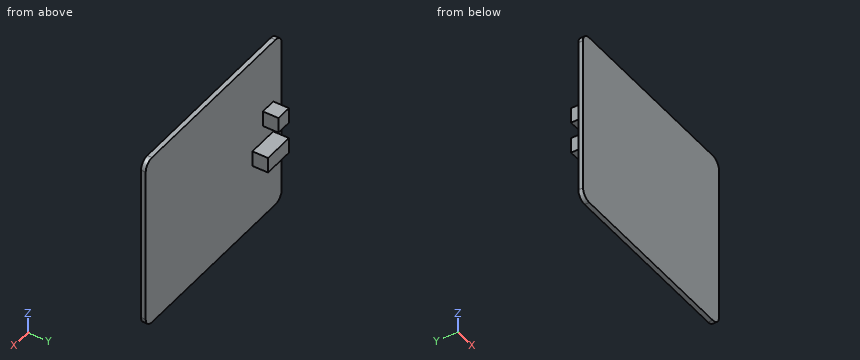
from build123d import *

# Parameters (mm, degrees)
SKETCH1_W           = 65
SKETCH1_H           = 56.6
BOSS_EXTRUDE1_DEPTH = 1.5
FILLET1_R           = 3
SKETCH2_W           = 5
SKETCH2_H           = 5
SKETCH2_W_2         = 10
BOSS_EXTRUDE2_DEPTH = 5


with BuildPart() as part:
    # Sketch1 → Boss-Extrude1 (new body)
    with BuildSketch(Plane(origin=(0, 0, 0), x_dir=(1, 0, 0), z_dir=(0, 1, 0))):
        with Locations((32.5, 28.3)):
            Rectangle(SKETCH1_W, SKETCH1_H)
    extrude(amount=BOSS_EXTRUDE1_DEPTH)

    # Fillet1
    fillet1_edges = [part.edges().sort_by_distance(p)[0] for p in [
        (0, 0.75, -56.6),
        (65, 0.75, -56.6),
        (65, 0.75, 0),
        (0, 0.75, 0),
    ]]
    fillet(fillet1_edges, radius=FILLET1_R)

    # Sketch2 → Boss-Extrude2 (add)
    with BuildSketch(Plane(origin=(0, 1.5, 0), x_dir=(1, 0, 0), z_dir=(0, 1, 0))):
        with Locations((6.5, 23)):
            Rectangle(SKETCH2_W, SKETCH2_H)
        with Locations((9, 33.3)):
            Rectangle(SKETCH2_W_2, SKETCH2_H)
    extrude(amount=BOSS_EXTRUDE2_DEPTH)


solid = part.part
Work out the finished part from the listing and answer in its coordinate system (mm). Give positions to 0.01 mm unless a question says otherwise; leave off trailing zeros. Write each loop counter-clockwise with the first axis right and the second up, starting at its lowest first coordinate (ties: lowest second). Pieces come first, ordered by that corner, then holes.
Q1. Given pin 1 (1.5 mm diameter, centred on y = 3, z = -34, fed in from +X); pin 2 (2.5 mm diameter, centred on x = 6, y = 3.5, fed in from -Z); pin 3 (12 mm diameter, centred on x = 50.5, z = -23.5, fed in from +Y), each flat-ended and moving along its own axis, determine where each tip first touches the part or whether it passes through.
Answer:
pin 1: stops at x = 14
pin 2: stops at z = -35.8
pin 3: stops at y = 1.5
Q2. The part is cut by section C-C on x = 7.5. Give the vertices of the cut face in (y, z).
Answer:
outline: (0, -56.6) - (1.5, -56.6) - (1.5, -35.8) - (6.5, -35.8) - (6.5, -30.8) - (1.5, -30.8) - (1.5, -25.5) - (6.5, -25.5) - (6.5, -20.5) - (1.5, -20.5) - (1.5, 0) - (0, 0) - close
Q3. Straight lines are drawn through the part: L1, parallel to Y at x = 59.5, z = -23.5; L2, parallel to Z at x = 11, y = 3; L3, parallel to Z at x = 6, y = 4. For each, find the intervals that lie inside material, in ascending order.
Answer:
L1: y = 0 to 1.5
L2: z = -35.8 to -30.8
L3: z = -35.8 to -30.8, -25.5 to -20.5
Q4. The part is cut by section A-A on y = 4.25. Give the vertices of the cut face in (x, z), and give its area (3 significant figures).
Answer:
outline: (4, -35.8) - (14, -35.8) - (14, -30.8) - (4, -30.8) - close; (4, -25.5) - (9, -25.5) - (9, -20.5) - (4, -20.5) - close
area: 75.0 mm2
Q5. The part is cut by section B-B on z = -33. Give the vertices of the cut face in (x, y), and give its area (4 significant figures).
Answer:
outline: (0, 0) - (65, 0) - (65, 1.5) - (14, 1.5) - (14, 6.5) - (4, 6.5) - (4, 1.5) - (0, 1.5) - close
area: 147.5 mm2
Q6. The part is cut by section D-D on z = -24. Give the vertices of the cut face in (x, y), and give its area (4 significant figures).
Answer:
outline: (0, 0) - (65, 0) - (65, 1.5) - (9, 1.5) - (9, 6.5) - (4, 6.5) - (4, 1.5) - (0, 1.5) - close
area: 122.5 mm2
